Can you work these out from the model? Positions are in its coordinate system, mm. A direction names the side the tool comes from. Give positions to 0.01 mm unless a question says otherwise; leave off trailing zeros. Loops run counter-clockwise (first coordinate to the right, second up) from the corner with the lowest first, then second, coordinate; pieces in that order, holes last. Notation, with made-up numbers: (12, 28) - (32, 28) arc R23 cw to (32, 55) - close; hole circle Ø1 at (-24.75, 40). An arc over 180 degrees is marked (long way). Answer in a Markdown table with one row per item.
from build123d import *

# Parameters (mm, degrees)
F0_R     = 6.35
F1_DEPTH = 31.75
F2_T     = 3.175


# Not quite as in the source:
# - a shell that OpenCascade refuses in one call is made with other operations: the cavity is built on its own and cut out


with BuildPart() as f1:
    # F0 (on Front) → F1 (new body)
    with BuildSketch(Plane.XZ):
        with BuildLine():
            Line((1066.8, 0), (76.2, 0))
            Line((76.2, 0), (76.2, 31.75))
            ThreePointArc((76.2, 31.75), (68.7605122421, 49.7105122421), (50.8, 57.15))
            Line((50.8, 57.15), (25.4, 57.15))
            ThreePointArc((25.4, 57.15), (7.4394877579, 49.7105122421), (0, 31.75))
            Line((0, 31.75), (0, 0))
            ThreePointArc((0, 0), (14.8789755157, -35.9210244843), (50.8, -50.8))
            Line((50.8, -50.8), (1066.8, -50.8))
            Line((1066.8, -50.8), (1066.8, 0))
        make_face()
        with Locations((577.85, -20.32)):
            Circle(F0_R, mode=Mode.SUBTRACT)
        with Locations((38.1, 35.56)):
            Circle(F0_R, mode=Mode.SUBTRACT)
    extrude(amount=F1_DEPTH)

    # F2: shell of thickness 3.175, made by hand


with BuildPart() as f2_core1:
    # F2_t2: copy of F1
    add(f1.part)

    # the walls: a layer under each face that stays
    f2_faces = [f2_core1.faces().sort_by_distance(p)[0] for p in [
        (571.5, -15.875, 0),
        (38.1, -15.875, 57.15),
        (0, -15.875, 15.875),
        (14.8789755157, -15.875, -35.9210244843),
        (558.8, -15.875, -50.8),
        (177.8, 0, -32.8083333333),
        (177.8, -31.75, -32.8083333333),
    ]]
    thicken(f2_faces, amount=-F2_T, mode=Mode.SUBTRACT)


with BuildPart() as f1_1:
    add(f1.part)

    # what is left inside the walls is the cavity
    f2_cavity = [f2_core1.part.solids().sort_by_distance(p)[0] for p in [
        (533.4, -28.54325, -12.7),
    ]]
    add(f2_cavity, mode=Mode.SUBTRACT)


solid = f1_1.part
Q1. If I drill on line 1 (Z direction, x = 444.5, y = -28) (3 decimals); line 2 (Y direction, x = 321.5, z = -36) (3 decimals); line 3 (Z direction, x = 577.85, y = -30.85), over which ranges is the centre line in solid material (lowest first)? Write a range as [from, to].
Checked values:
| item | result |
|---|---|
| line 1 | z = [-50.8, -47.625], [-3.175, 0] |
| line 2 | y = [-31.75, -28.575], [-3.175, 0] |
| line 3 | z = [-50.8, -26.67], [-13.97, 0] |
Q2. For pin 1 (1 mm diameter, centred on y = -29.5, z = 8.5, fed in from +X); pin 2 (3 mm diameter, centred on y = -28, z = -11.5, fed in from -X); pin 3 (12.5 mm diameter, centred on x = 35.5, y = -16.5, fed in from -Z), each with a flat end and sliding along its axis, tell me the tip position at first contact or that it passes through.
Checked values:
| item | result |
|---|---|
| pin 1 | stops at x = 76.2 |
| pin 2 | stops at x = 0.99 |
| pin 3 | stops at z = -49.99 |
Q3. Imagine slicing it at C-C, the plane z = 13. Write out the boundary of the cut face in (x, y) (3 decimals).
Checked values:
| item | result |
|---|---|
| outline | (0, -31.75) - (76.2, -31.75) - (76.2, -28.575) - (3.175, -28.575) - (3.175, -3.175) - (76.2, -3.175) - (76.2, 0) - (0, 0) - close |
Q4. Imagine slicing it at A-A, the plane y = -9. Write out the boundary of the cut face in (x, z) (3 decimals).
Checked values:
| item | result |
|---|---|
| outline | (0, 0) arc R50.8 ccw to (50.8, -50.8) - (1066.8, -50.8) - (1066.8, -47.625) - (50.8, -47.625) arc R47.625 cw to (3.175, 0) - (3.175, 31.75) - (0, 31.75) - close; (25.4, 53.975) - (50.8, 53.975) - (50.8, 57.15) - (25.4, 57.15) - close; (76.2, -3.175) - (1066.8, -3.175) - (1066.8, 0) - (76.2, 0) - close |
Q5. Imagine slicing it at B-B, the plane x = 613.5. Write out the boundary of the cut face in (y, z) (3 decimals).
Checked values:
| item | result |
|---|---|
| outline | (-31.75, -50.8) - (0, -50.8) - (0, 0) - (-31.75, 0) - close; hole (-28.575, -47.625) - (-3.175, -47.625) - (-3.175, -3.175) - (-28.575, -3.175) - close |
Q6. If we mould it in two halves opening along Z, with no side actions, what happens to faces 1 (the face through (1066.8, -3, -26)), 2 (the face through (68.96, -30.14, 49.51)), 3 (the face through (552, -16, -47.625))? For each: released by +Z, released by -Z, zero draft, split by the parting line, or undercut.
Checked values:
| item | result |
|---|---|
| face 1 | zero draft |
| face 2 | released by +Z |
| face 3 | undercut |
Q7. On a 3-axis mill with a long thin cutter (end or side, diameter ignored), from which of +Z, -Z, +X, -X, +Y, -Y can I reach the whole of each face in a straight line? I mean faces 4 (the face through (578, -16, 0)), 5 (the face through (578, -16, -3.175)), 6 (the face through (3.175, -16, 16)). Say none if no direction works.
Checked values:
| item | result |
|---|---|
| face 4 | +Z, +X, +Y, -Y |
| face 5 | +X |
| face 6 | +Z, +X |
